Input: part model. Units: mm. Frame: model coordinates. Face numbers are marked on the shaded views. A direction names the side the tool comes from. Round coordinates to 2 decimals unless told otherwise and drop trailing zeros. Write each loop counter-clockwise with the first axis right and the second up, starting at its lowest first coordinate (ties: lowest second). Pieces come first, ordered by that corner, then holes. Notation, with made-up numbers: M 22,39 L 69,39 A13 ccw 69,64 Z; hole C 2,12.5 d10. An arc over 180 degrees is marked long. Write each question's results on one line, items separated by ' | '. Start each with the question number.
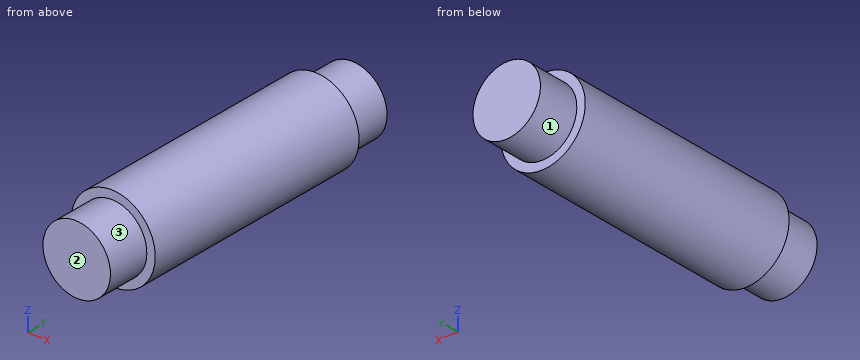
```python
from build123d import *

# Parameters (mm, degrees)
SKETCH1_W           = 2.5
SKETCH1_H           = 14
SKETCH2_R           = 2
BOSS_EXTRUDE1_DEPTH = 2.5
BOSS_EXTRUDE2_START = 2.5
SKETCH3_R           = 2
BOSS_EXTRUDE2_DEPTH = 2.5


with BuildPart() as part:
    # Sketch1 → Revolve-Thin1 (revolve)
    with BuildSketch(Plane.XY, mode=Mode.PRIVATE) as revolve_thin1_sk:
        with Locations((-1.25, 7)):
            Rectangle(SKETCH1_W, SKETCH1_H)
    revolve(revolve_thin1_sk.sketch.rotate(Axis((0, 0, 0), (0, 1, 0)), 270), axis=Axis((0, 0, 0), (0, 1, 0)))

    # Sketch2 → Boss-Extrude1 (add)
    with BuildSketch(Plane(origin=(0, 14, 0), x_dir=(1, 0, 0), z_dir=(0, 1, 0))):
        with Locations(Location((0, 0, 0), (0, 0, 90))):
            Circle(SKETCH2_R)
    extrude(amount=BOSS_EXTRUDE1_DEPTH)

    # Sketch3 → Boss-Extrude2 (add)
    with BuildSketch(Plane(origin=(0, 0, 0), x_dir=(-1, 0, 0), z_dir=(0, -1, 0)).offset(BOSS_EXTRUDE2_START)):
        with Locations(Location((0, 0, 0), (0, 0, 90))):
            Circle(SKETCH3_R)
    extrude(amount=-BOSS_EXTRUDE2_DEPTH)


solid = part.part
```
1. Line query: L1, parallel to Z at x = 0.1, y = 7.5; L2, parallel to Y at x = -1.8, z = -1.05; L3, parallel to Z at x = -1.5, y = 0.5. Output: solid intervals per line, ascending. Write a range as from..to.
2. Cut plane B-B on z = 0. Output: boundary loops of the cut face in (x, y), and give its area (3 significant figures).
3. Access query for the marked faces 1, 2 and 3. Directions: +Z, -Z, +X, -X, +Y, -Y. A direction counts if a zero-diameter tool reaches every point of the face in a straight line with its end or side. Return the directions, or none.
4. Cut plane C-C on y = 2. Output: boundary loops of the cut face in (x, z), and give its area (3 significant figures).
5. Cut plane A-A on x = 0. Output: boundary loops of the cut face in (y, z), and give its area (3 significant figures).
6. Contact query for a flat-ended pin moving along its axis: P1, Ø2, axis at y = 7, z = -1.5, coming from the -X side. Output: stop coordinate, or through.
Answers follow:
1) L1: z = -2.5..2.5 | L2: y = 0..14 | L3: z = -2..2
2) outline: M -2.5,0 L -2,0 L -2,-2.5 L 2,-2.5 L 2,0 L 2.5,0 L 2.5,14 L 2,14 L 2,16.5 L -2,16.5 L -2,14 L -2.5,14 Z | area: 90.0 mm2
3) face 1: +Y | face 2: +Z, -Z, +X, -X, -Y | face 3: -Y
4) outline: C 0,0 d5 | area: 19.6 mm2
5) outline: M -2.5,-2 L 0,-2 L 0,-2.5 L 14,-2.5 L 14,-2 L 16.5,-2 L 16.5,2 L 14,2 L 14,2.5 L 0,2.5 L 0,2 L -2.5,2 Z | area: 90.0 mm2
6) P1: stops at x = -2.45
